```python
from build123d import *


with BuildPart() as cono001:
    # Cone001 → Cone001 (revolve)
    with BuildSketch(Plane(origin=(0, 0, 1), x_dir=(1, 0, 0), z_dir=(0, -1, 0))):
        Polygon((0, 0), (19, 0), (29, 80), (0, 80), align=None)
    revolve(axis=Axis((0, 0, 1), (0, 0, 1)))


with BuildPart() as cut:
    # Cone → Cone (revolve)
    with BuildSketch(Plane.XZ):
        Polygon((0, 0), (20, 0), (30, 80), (0, 80), align=None)
    revolve(axis=Axis((0, 0, 0), (0, 0, 1)))

    # Cut: cut Cono001
    add(cono001.part, mode=Mode.SUBTRACT)


solid = cut.part
```
Geometry: final body of the model. Coordinates: model frame, mm. A direction names the side the tool comes from. Coordinates: 2 decimals unless noted, no trailing zeros. Order: outer loops, then holes, each group sorted by start corner. A loop starts at its lowest first (then second) coordinate and runs counter-clockwise, first axis right, second up.
Item 1: Draft query along X for faces 3 (the face through (23.912, 7.53, 40.56)), 4 (the face through (-16, 25, 80)), 5 (the face through (22.9, 7.21, 41.05)). Return one class per face: released by +X, released by -X, zero draft, split by the parting line, or undercut.
Answer:
face 3: split by the parting line
face 4: zero draft
face 5: undercut
Item 2: Access query for faces 1 (the face through (0, 0, 0)), 2 (the face through (0, 0, 1)). Directions: +Z, -Z, +X, -X, +Y, -Y. A direction counts if a zero-diameter tool reaches every point of the face in a straight line with its end or side. Return the directions, or none.
Answer:
face 1: -Z, +X, -X, +Y, -Y
face 2: +Z
Item 3: Material intervals for line 1 along Y through (x, z) = (-18, 5); line 2 along Y through (x, z) = (2, 29); line 3 along X through (y, z) = (10, 52.5), sorted ascending.
Answer:
line 1: y = -10.07 to -7.5, 7.5 to 10.07
line 2: y = -23.54 to -22.41, 22.41 to 23.54
line 3: x = -24.61 to -23.39, 23.39 to 24.61
Item 4: Section query D-D (z = 75). Output: boundary loops of the cut face in (x, y) (3 decimals).
Answer:
outline: circle Ø58.75 at (0, 0); hole circle Ø56.5 at (0, 0)
Item 5: Contact query for flat-ended pins moving along their axis: P1, Ø2, axis at x = -18.5, z = 42.5, coming from the -Y side; P2, Ø2, axis at y = -1.5, z = 68, coming from the +X side; P3, Ø4, axis at x = 16.5, z = 57, coming from the +Y side. Output: stop coordinate, or through.
Answer:
P1: stops at y = -18.3
P2: stops at x = 28.59
P3: stops at y = 22.96
Item 6: Section query A-A (y = 0). Output: boundary loops of the cut face in (x, z) (3 decimals), then the cut area to 3 significant figures.
Answer:
outline: (-30, 80) - (-20, 0) - (20, 0) - (30, 80) - (28.875, 80) - (19, 1) - (-19, 1) - (-28.875, 80) - close
area: 218 mm2
Item 7: Section query C-C (z = 14). Output: boundary loops of the cut face in (x, y) (3 decimals), then the cut area to 3 significant figures.
Answer:
outline: circle Ø43.5 at (0, 0); hole circle Ø41.25 at (0, 0)
area: 150 mm2
